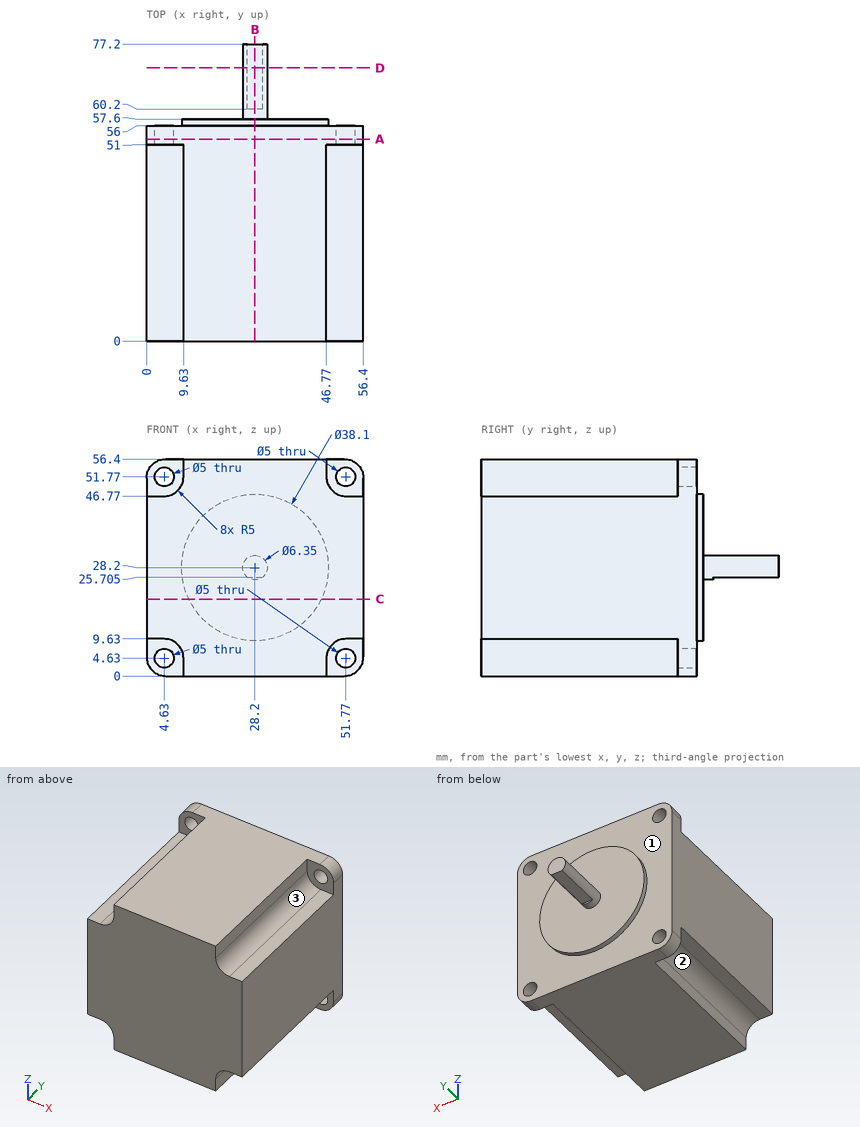
For this review, use the dimensioned drawing (mm, ordinates from the lowest corner) and the shaded views. A direction names the side the tool comes from. Round coordinates to 2 decimals unless told otherwise and drop trailing zeros. Loops run counter-clockwise (first coordinate to the right, second up) from the corner with the lowest first, then second, coordinate; pieces in that order, holes last. Notation, with made-up numbers: M 80.5,22.25 L 122.5,22.25 A19 cw 122.5,49.25 Z; hole C 26.25,-17 d1. An arc over 180 degrees is marked long. Answer as a JSON object with one key per item and string values.
(1) Take a section at A-A on y = 52.5. Give the boundary of the cut face in (x, z), and give its area (3 significant figures).
Resolved:
{"outline": "M 0,5 A5 ccw 5,0 L 51.4,0 A5 ccw 56.4,5 L 56.4,51.4 A5 ccw 51.4,56.4 L 5,56.4 A5 ccw 0,51.4 Z; hole C 4.63,4.63 d5; hole C 4.63,51.77 d5; hole C 51.77,4.63 d5; hole C 51.77,51.77 d5", "area": "3,080 mm²"}
(2) Tool access review of the marked faces 1, 2 and 3: name each direction out of +Z, -Z, +X, -X, +Y, -Y from which nothing blocks a thin tool from reaching the whole face with its end or side.
Resolved:
{"face 1": "+Y", "face 2": "-Z, -X, -Y", "face 3": "+Z, +X, -Y"}
(3) Take a section at B-B on x = 28.2. Give the boundary of the cut face in (y, z) (3 decimals).
Resolved:
{"outline": "M 0,0 L 56,0 L 56,9.15 L 57.6,9.15 L 57.6,25.025 L 60.2,25.025 L 60.2,25.705 L 77.2,25.705 L 77.2,31.375 L 57.6,31.375 L 57.6,47.25 L 56,47.25 L 56,56.4 L 0,56.4 Z"}
(4) Take a section at C-C on z = 20. Give the boundary of the cut face in (x, y).
Resolved:
{"outline": "M 0,0 L 56.4,0 L 56.4,56 L 45.39,56 L 45.39,57.6 L 11.01,57.6 L 11.01,56 L 0,56 Z"}
(5) Take a section at D-D on y = 71. Give the boundary of the cut face in (x, z) (3 decimals).
Resolved:
{"outline": "M 26.236,25.705 L 30.164,25.705 A3.175 ccw long Z"}
(6) To check wall thickness, follow line 1 along X through (y, z) = (53.15, 51.77); line 2 along X through (y, z) = (53, 4). State the ranges of each line that lie inside material, in increasing order.
Resolved:
{"line 1": "0.01 to 2.13, 7.13 to 49.27, 54.27 to 56.39", "line 2": "0.1 to 2.21, 7.05 to 49.35, 54.19 to 56.3"}
(7) Clearance check with flat-ended pins moving along their axes: P1, Ø5, axis at x = 3, z = 51.5, coming from the -Y side; P2, Ø2.5, axis at y = 21.5, z = 55, coming from the +X side; P3, Ø1.4, axis at x = 54, y = 14.5, coming from the -Z side. State where each tip first meets the part, or that it passes through.
Resolved:
{"P1": "y = 51", "P2": "x = 46.77", "P3": "z = 9.63"}
